Check sheet for the drawn part. Datum: minimum x, y, z corner. Units: mm. A direction names the side the tool comes from. Coordinates: 2 decimals unless noted, no trailing zeros. Loops run counter-clockwise (first coordinate to the right, second up) from the corner with the lowest first, then second, coordinate; pieces in that order, holes last. Notation, with made-up numbers: M -29.5,80.5 L -8.5,80.5 A22 ccw -8.5,86.5 Z; hole C 1.5,-2 d4. An arc over 180 degrees is marked long. Use CSV: the item, a comma, the result in double quotes. Start each with the question number.
(1) Section check B-B on z = 1.5. Record the cut outline in (x, y), and give its area (3 significant figures).
(2) Section check C-C on x = 13.5. Record the cut outline in (y, z).
(3) Set-up check for the marked faces 1, 2, 3, 4 and 5: record each of +Z, -Z, +X, -X, +Y, -Y from which the full face is reachable in a straight line by a thin tool's end or side.
(4) Section check A-A on y = 5.75. Record the cut outline in (x, z), and give its area (3 significant figures).
(5) Go/stop test with flat-tipped pins: pin 1 Ø0.9 at (x, z) = (21, 2) entering from +Y; pin 2 Ø1.5 at (x, z) = (34.5, 2) entering from +Y. Record where each tip stops, or that it passes through.
(6) Draft check along X on the marked faces 6, 7 and 8. Enter one of: pulls with the +X half, pulls with the -X half, needs draft (parallel to the pull), parting line crosses it, or undercut.
(7) Section check D-D on y = 2.5. Record the cut outline in (x, z).
(8) Scan lines: line 1 (Y direction, x = 26, z = 1.15); line 2 (X direction, y = 6, z = 2.75); line 3 (Y direction, x = 4, z = 2.45). Record each from-to range of solid material in increasing order.
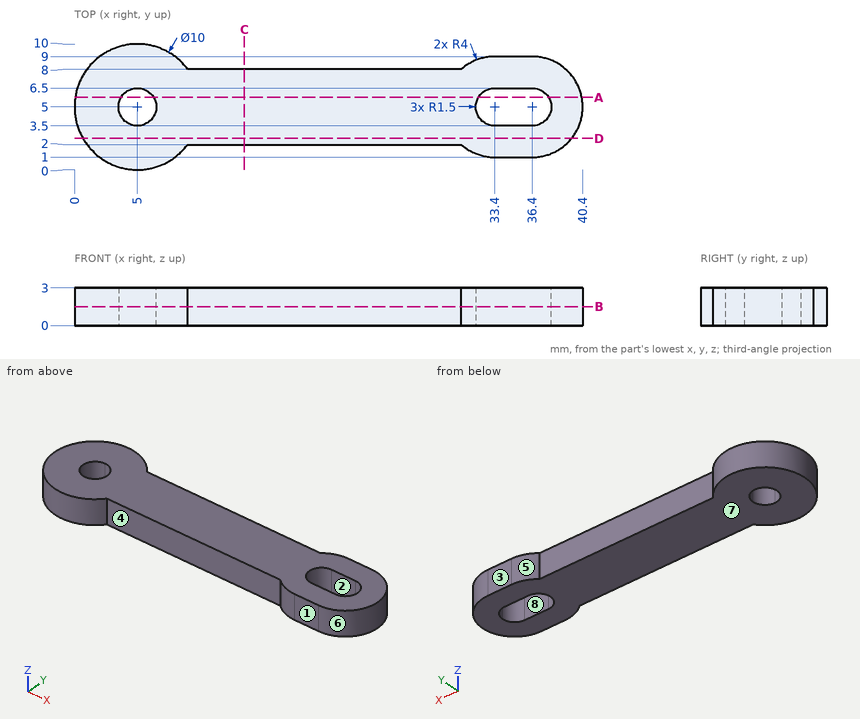
Outcome:
1,outline,"M 9,2 L 30.75,2 A4 ccw 33.4,1 L 36.4,1 A4 ccw 36.4,9 L 33.4,9 A4 ccw 30.75,8 L 9,8 A5 ccw long Z; hole C 5,5 d3; hole M 33.4,3.5 L 36.4,3.5 A1.5 ccw 36.4,6.5 L 33.4,6.5 A1.5 ccw Z"
1,area,"250 mm²"
2,outline,"M 2,0 L 8,0 L 8,3 L 2,3 Z"
3,face 1,"+Z, -Z, +X, -Y"
3,face 2,"+Z, -Z"
3,face 3,"+Z, -Z, +X, +Y"
3,face 4,"+Z, -Z, -Y"
3,face 5,"+Z, -Z, +Y"
4,outline,"M 0.06,0 L 3.7,0 L 3.7,3 L 0.06,3 Z; M 6.3,0 L 32.1,0 L 32.1,3 L 6.3,3 Z; M 37.7,0 L 40.33,0 L 40.33,3 L 37.7,3 Z"
4,area,"96.2 mm²"
5,pin 1,"stops at y = 8"
5,pin 2,"stops at y = 9"
6,face 6,"pulls with the +X half"
6,face 7,"needs draft"
6,face 8,"undercut"
7,outline,"M 0.67,0 L 39.52,0 L 39.52,3 L 0.67,3 Z"
8,line 1,"y = 2 to 8"
8,line 2,"x = 0.1 to 3.88, 6.12 to 32.28, 37.52 to 40.27"
8,line 3,"y = 0.1 to 3.88, 6.12 to 9.9"
